from build123d import *

# Parameters (mm, degrees)
SKETCH_1_R          = 7
EXTRUDE_1_DEPTH     = 22.5
SKETCH_2_R          = 5.5
SKETCH_2_R_2        = 5
EXTRUDE_2_DEPTH     = 74
SKETCH_3_R          = 7
EXTRUDE_3_DEPTH     = 12.5
SKETCH_4_R          = 4
EXTRUDE_4_DEPTH     = 8.5
SKETCH_5_R          = 2
CUT_EXTRUDE_1_DEPTH = 50
SKETCH_6_R          = 10
SKETCH_6_W          = 12
SKETCH_6_H          = 12
CUT_EXTRUDE_2_DEPTH = 110.448618082
SKETCH_7_W          = 3.2
SKETCH_7_H          = 12
CUT_EXTRUDE_3_DEPTH = 13
SKETCH_8_R          = 1.6
CUT_EXTRUDE_4_DEPTH = 119.263477033
SKETCH_9_R          = 2.5
CUT_EXTRUDE_5_DEPTH = 5
SKETCH_10_R         = 2.5
CUT_EXTRUDE_6_DEPTH = 5


with BuildPart() as part:
    # 草图1 → 凸台-拉伸1 (new body)
    with BuildSketch(Plane.XY):
        with Locations(Location((0, 0, 0), (0, 0, 180))):
            Circle(SKETCH_1_R)
    extrude(amount=EXTRUDE_1_DEPTH)

    # 草图2 → 凸台-拉伸2 (add)
    with BuildSketch(Plane.XY.offset(22.5)):
        Circle(SKETCH_2_R)
        Circle(SKETCH_2_R_2, mode=Mode.SUBTRACT)
    extrude(amount=EXTRUDE_2_DEPTH)

    # 草图3 → 凸台-拉伸3 (add)
    with BuildSketch(Plane.XY.offset(96.5)):
        with Locations(Location((0, 0, 0), (0, 0, 180))):
            Circle(SKETCH_3_R)
    extrude(amount=EXTRUDE_3_DEPTH)

    # 草图4 → 凸台-拉伸4 (add)
    with BuildSketch(Plane.XY.offset(109)):
        Circle(SKETCH_4_R)
    extrude(amount=EXTRUDE_4_DEPTH)

    # 草图5 → 切除-拉伸1 (cut)
    with BuildSketch(Plane.XY.offset(117.5)):
        Circle(SKETCH_5_R)
    extrude(amount=-CUT_EXTRUDE_1_DEPTH, mode=Mode.SUBTRACT)

    # 草图6 → 切除-拉伸2 (cut, through all)
    with BuildSketch(Plane.XY.offset(109)):
        Circle(SKETCH_6_R)
        Rectangle(SKETCH_6_W, SKETCH_6_H, mode=Mode.SUBTRACT)
    extrude(amount=-CUT_EXTRUDE_2_DEPTH, mode=Mode.SUBTRACT)

    # 草图7 → 切除-拉伸3 (cut)
    with BuildSketch(Plane(origin=(0, 0, 0), x_dir=(-1, 0, 0), z_dir=(0, 0, -1))):
        Rectangle(SKETCH_7_W, SKETCH_7_H)
    extrude(amount=-CUT_EXTRUDE_3_DEPTH, mode=Mode.SUBTRACT)

    # 草图8 → 切除-拉伸4 (cut, through all)
    with BuildSketch(Plane(origin=(6, 0, 0), x_dir=(0, 0, -1), z_dir=(1, 0, 0))):
        with Locations((-5, 0)):
            Circle(SKETCH_8_R)
    extrude(amount=-CUT_EXTRUDE_4_DEPTH, mode=Mode.SUBTRACT)

    # 草图9 → 切除-拉伸5 (cut)
    with BuildSketch(Plane(origin=(0, 6, 0), x_dir=(1, 0, 0), z_dir=(0, 1, 0))):
        with Locations(Location((0, -18, 0), (0, 0, 270))):
            Circle(SKETCH_9_R)
    extrude(amount=-CUT_EXTRUDE_5_DEPTH, mode=Mode.SUBTRACT)

    # 草图10 → 切除-拉伸6 (cut)
    with BuildSketch(Plane(origin=(0, 6, 0), x_dir=(1, 0, 0), z_dir=(0, 1, 0))):
        with Locations(Location((0, -101, 0), (0, 0, 270))):
            Circle(SKETCH_10_R)
    extrude(amount=-CUT_EXTRUDE_6_DEPTH, mode=Mode.SUBTRACT)


solid = part.part
Model file for the job. Use its own axes, mm. A direction names the side the tool comes from. Coordinates: 2 decimals unless noted, no trailing zeros. Write each loop counter-clockwise with the first axis right and the second up, starting at its lowest first coordinate (ties: lowest second). Pieces come first, ordered by that corner, then holes. Notation, with made-up numbers: (29.25, 73) - (35.25, 73) arc R29 cw to (35.25, 107) - close; hole circle Ø9 at (31, -15). An arc over 180 degrees is marked (long way). Write each question's results on one line, items separated by ' | '. Start each with the question number.
1) Cut at C-C (z = 101). Write the cut outline in (x, y), then the cut area to 3 significant figures.
2) Mould opens along X. For faces 1 (the face through (-0.867, -3.905, 113.19)), 2 (the face through (1.6, 1.2, 6.4)), 3 (the face through (-2, 6, 11)) say: pulls with the +X half, pulls with the -X half, needs draft (parallel to the pull), parting line crosses it, or undercut.
3) Cut at B-B (z = 8.5). Write the cut outline in (x, y).
4) 3-axis set-ups, long thin cutter, end or side, ignore diameter. For faces 4 (the face through (3, 5, 22.5)), 5 (the face through (-4.9, 5, 102.7)), 6 (the face through (0, 0, 13)), 7 (the face through (0, 1, 18)): which of +Z, -Z, +X, -X, +Y, -Y reach the whole face in a straight line?
5) Cut at D-D (y = 0). Count the separate pieces of the cut face and the enclosed holes in it, then the cut area to 3 significant figures.
6) Probe line 1 along Z through (x, y) = (4.5, -0.25); line 2 along Y through (x, z) = (-3.5, 5); line 3 along X through (y, z) = (2.5, 18). List the from-to ranges inside material, lowest first. Write a range as from..to.
7) Flat gauge pins, fed straight in: P1, Ø6.5, axis at x = 0, y = 0, coming from the -Z side; P2, Ø4, axis at y = 4.5, z = 43.5, coming from the +X side; P3, Ø6, axis at y = 4, z = 79.5, coming from the -X side; P4, Ø1.5, axis at x = -3, z = 91.5, coming from the +Y side. Where does each tip first touch, or does it go through?
Returned:
1) outline: (-6, -3.61) arc R7 ccw to (-3.61, -6) - (3.61, -6) arc R7 ccw to (6, -3.61) - (6, 3.61) arc R7 ccw to (3.61, 6) - (2.5, 6) - (2.5, 1) - (1.73, 1) arc R2 cw (long way) to (-1.73, 1) - (-2.5, 1) - (-2.5, 6) - (-3.61, 6) arc R7 ccw to (-6, 3.61) - close | area: 99.3 mm^2
2) face 1: parting line crosses it | face 2: undercut | face 3: needs draft
3) outline: (-6, -3.61) arc R7 ccw to (-3.61, -6) - (-1.6, -6) - (-1.6, 6) - (-3.61, 6) arc R7 ccw to (-6, 3.61) - close; (1.6, -6) - (3.61, -6) arc R7 ccw to (6, -3.61) - (6, 3.61) arc R7 ccw to (3.61, 6) - (1.6, 6) - close
4) face 4: none | face 5: +Z, -Z, -X, +Y | face 6: -Z, +Y, -Y | face 7: +Y
5) separate pieces: 3 | enclosed holes: 0 | area: 408 mm^2
6) line 1: 0..3.42, 6.58..22.5, 96.5..109 | line 2: -6..-1.6, 1.6..6 | line 3: -6..-2.5, 2.5..6
7) P1: z = 0 | P2: x = 4.9 | P3: x = -5.41 | P4: y = 5.02
